```python
from build123d import *

# Parameters (mm, degrees)
F0_W     = 101.6
F0_H     = 50.8
F1_DEPTH = 25.4
F2_R     = 6.35
F3_DEPTH = 25.401
F4_W     = 12.7
F4_H     = 25.4
F6_W     = 8.301848
F6_H     = 6.35
F8_R     = 1.27
F9_SIZE  = 2.54


with BuildPart() as f1:
    # F0 (on Front) → F1 (new body)
    with BuildSketch(Plane.XZ):
        Rectangle(F0_W, F0_H)
    extrude(amount=F1_DEPTH)

    # F2 (on face) → F3 (cut, through all)
    with BuildSketch(Plane.XZ.offset(25.4)):
        with Locations((-38.1, 12.7)):
            Circle(F2_R)
        with Locations((-38.1, -12.7)):
            Circle(F2_R)
        with Locations((38.1, 12.7)):
            Circle(F2_R)
        with Locations((38.1, -12.7)):
            Circle(F2_R)
    extrude(amount=-F3_DEPTH, mode=Mode.SUBTRACT)

    # F4 (on Top) → F5 (revolve)
    with BuildSketch(Plane.XY):
        with Locations((6.35, -38.1)):
            Rectangle(F4_W, F4_H)
    revolve(axis=Axis((0, -38.1, 0), (0, 1, 0)))

    # F6 (on Top) → F7 (revolve, cut)
    with BuildSketch(Plane.XY):
        with Locations((-14.310924, -38.735)):
            Rectangle(F6_W, F6_H)
    revolve(axis=Axis((0, -40.756147, 0), (0, -1, 0)), mode=Mode.SUBTRACT)

    # F8
    f8_edges = [f1.edges().sort_by_distance(p)[0] for p in [
        (-12.7, -25.4, 0),
        (10.16, -35.56, 0),
        (10.16, -41.91, 0),
    ]]
    fillet(f8_edges, radius=F8_R)

    # F9
    f9_edges = [f1.edges().sort_by_distance(p)[0] for p in [
        (0, -25.4, 25.4),
        (-50.8, -25.4, 0),
        (0, -25.4, -25.4),
        (50.8, -25.4, 0),
    ]]
    chamfer(f9_edges, length=F9_SIZE)


solid = f1.part
```
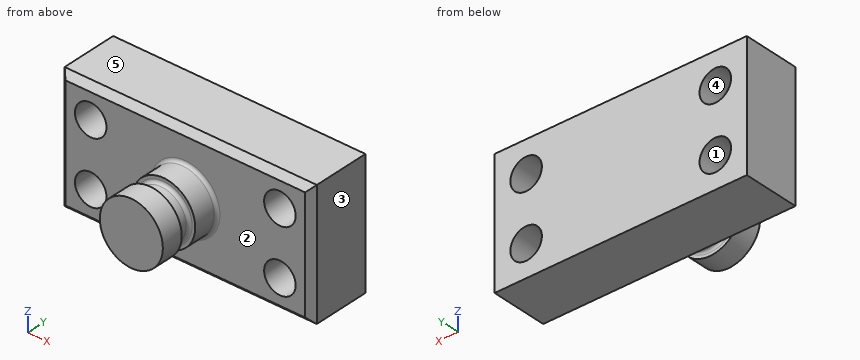
Geometry: final body of the model. Coordinates: model frame, mm. Face numbers are marked on the shaded views. A direction names the side the tool comes from. Round coordinates to 2 decimals unless told otherwise and drop trailing zeros. Loops run counter-clockwise (first coordinate to the right, second up) from the corner with the lowest first, then second, coordinate; pieces in that order, holes last. Notation, with made-up numbers: (28, 89.25) -> (57, 89.25) arc R31 ccw to (57, 125.25) -> close; hole circle Ø2 at (66, 14.5). An arc over 180 degrees is marked (long way). Use one line per item in the form item = value. Start each with the question number.
1) Draft query along X for the marked faces 3, 4 and 5. Return one class per face: released by +X, released by -X, zero draft, split by the parting line, or undercut.
2) Section A-A on y = -14.5. Output: boundary loops of the cut face in (x, z), then the cut area to 3 significant figures.
3) Section C-C on z = 0. Output: boundary loops of the cut face in (x, y).
4) Line query: L1, parallel to Z at x = 38, y = -18; L2, parallel to X at y = -24, z = 9.5; L3, parallel to X at y = -21, z = 13. Output: solid intervals per line, ascending.
5) Access query for the marked faces 1 and 2. Directions: +Z, -Z, +X, -X, +Y, -Y. A direction counts if a zero-diameter tool reaches every point of the face in a straight line with its end or side. Return the directions, or none.
6) First-contact query: P1, Ø20.5, axis at x = 38.1, z = 12.7, coming from the +Y side; P2, Ø5, axis at y = -25.5, z = 15.5, coming from the -X side; P3, Ø16.5, axis at x = 38.1, z = -12.7, coming from the -Y side; P4, Ø4, axis at y = -43.5, z = 10.5, coming from the +X side. Flat tips, straight axial feed; report the tip coordinate or a pass-through.
7) Section D-D on x = 0. Output: boundary loops of the cut face in (y, z), then the cut area to 3 significant figures.
8) Section B-B on x = 38.1. Output: boundary loops of the cut face in (y, z), then the cut area to 3 significant figures.
Response:
q1.face_3 = released by +X
q1.face_4 = undercut
q1.face_5 = zero draft
q2.outline = (-50.8, -25.4) -> (50.8, -25.4) -> (50.8, 25.4) -> (-50.8, 25.4) -> close; hole circle Ø12.7 at (-38.1, -12.7); hole circle Ø12.7 at (-38.1, 12.7); hole circle Ø12.7 at (38.1, -12.7); hole circle Ø12.7 at (38.1, 12.7)
q2.area = 4,650 mm^2
q3.outline = (-50.8, -22.86) -> (-48.26, -25.4) -> (-13.97, -25.4) arc R1.27 cw to (-12.7, -26.67) -> (-12.7, -35.56) -> (-11.43, -35.56) arc R1.27 cw to (-10.16, -36.83) -> (-10.16, -40.64) arc R1.27 cw to (-11.43, -41.91) -> (-12.7, -41.91) -> (-12.7, -50.8) -> (12.7, -50.8) -> (12.7, -41.91) -> (11.43, -41.91) arc R1.27 cw to (10.16, -40.64) -> (10.16, -36.83) arc R1.27 cw to (11.43, -35.56) -> (12.7, -35.56) -> (12.7, -26.67) arc R1.27 cw to (13.97, -25.4) -> (48.26, -25.4) -> (50.8, -22.86) -> (50.8, 0) -> (-50.8, 0) -> close
q4.L1 = -25.4 to -19.05, -6.35 to 6.35, 19.05 to 25.4
q4.L2 = -49.66 to -43.58, -32.62 to 32.62, 43.58 to 49.66
q4.L3 = -50.8 to -44.44, -31.76 to 31.76, 44.44 to 50.8
q5.face_1 = +Y, -Y
q5.face_2 = -Y
q6.P1 = 0
q6.P2 = -50.66
q6.P3 = -25.4
q6.P4 = 9.44
q7.outline = (-50.8, -12.7) -> (-41.91, -12.7) -> (-41.91, -11.43) arc R1.27 cw to (-40.64, -10.16) -> (-36.83, -10.16) arc R1.27 cw to (-35.56, -11.43) -> (-35.56, -12.7) -> (-26.67, -12.7) arc R1.27 cw to (-25.4, -13.97) -> (-25.4, -22.86) -> (-22.86, -25.4) -> (0, -25.4) -> (0, 25.4) -> (-22.86, 25.4) -> (-25.4, 22.86) -> (-25.4, 13.97) arc R1.27 cw to (-26.67, 12.7) -> (-35.56, 12.7) -> (-35.56, 11.43) arc R1.27 cw to (-36.83, 10.16) -> (-40.64, 10.16) arc R1.27 cw to (-41.91, 11.43) -> (-41.91, 12.7) -> (-50.8, 12.7) -> close
q7.area = 1,900 mm^2
q8.outline = (-25.4, -22.86) -> (-22.86, -25.4) -> (0, -25.4) -> (0, -19.05) -> (-25.4, -19.05) -> close; (-25.4, -6.35) -> (0, -6.35) -> (0, 6.35) -> (-25.4, 6.35) -> close; (-25.4, 19.05) -> (0, 19.05) -> (0, 25.4) -> (-22.86, 25.4) -> (-25.4, 22.86) -> close
q8.area = 639 mm^2
